from build123d import *

# Parameters (mm, degrees)
SKETCH1_R           = 2.875
SKETCH1_R_2         = 7
BOSS_EXTRUDE1_DEPTH = 24.5875
SKETCH4_W           = 66.272407177
SKETCH4_H           = 27.800260981
CUT_EXTRUDE2_DEPTH  = 20
FILLET3_R           = 10
FILLET4_R           = 10
BOSS_EXTRUDE3_START = -1.5875
BOSS_EXTRUDE3_DEPTH = 1.5875
SKETCH7_R           = 7
CUT_EXTRUDE3_DEPTH  = 1.5875
CUT_EXTRUDE4_START  = -10
SKETCH8_R           = 3
SKETCH8_R_2         = 18.9
SKETCH8_R_3         = 2.875
SKETCH8_R_4         = 7
CUT_EXTRUDE4_DEPTH  = 10
SKETCH9_W           = 229.1070397
SKETCH9_H           = 361.266964835
SKETCH9_R           = 1.388229101
SKETCH9_R_2         = 1.483383261
SKETCH9_R_3         = 1.314910669
SKETCH9_R_4         = 1.248623853
SKETCH9_R_5         = 1.255629307
SKETCH9_R_6         = 1.53911217
CUT_EXTRUDE5_DEPTH  = 13
SKETCH10_W          = 29.988446547
SKETCH10_H          = 5
SKETCH10_H_2        = 5.75
CUT_EXTRUDE6_DEPTH  = 22
SKETCH11_R          = 5.236653548
CUT_EXTRUDE7_DEPTH  = 10
BOSS_EXTRUDE4_START = -1.59
BOSS_EXTRUDE4_DEPTH = 1.59
SKETCH13_R          = 7
CUT_EXTRUDE8_DEPTH  = 41
SKETCH14_W          = 61.491848917
SKETCH14_H          = 35.587491391
CUT_EXTRUDE9_DEPTH  = 20
FILLET5_R           = 10
SKETCH16_W          = 163.723031551
SKETCH16_H          = 22.872070304
CUT_EXTRUDE11_DEPTH = 35
FILLET6_R           = 10
SKETCH17_R          = 1.53911217
SKETCH17_R_2        = 1.255629307
SKETCH17_R_3        = 1.3
SKETCH17_R_4        = 1.314910669
SKETCH17_R_5        = 1.388229101
SKETCH17_R_6        = 1.5
CUT_EXTRUDE12_DEPTH = 42
CUT_EXTRUDE13_START = -30
SKETCH18_R          = 18.9
CUT_EXTRUDE13_DEPTH = 30
SKETCH19_R          = 7
BOSS_EXTRUDE5_DEPTH = 3.175


with BuildPart() as part:
    # Sketch1 → Boss-Extrude1 (new body)
    with BuildSketch(Plane(origin=(0, 0, 0), x_dir=(1, 0, 0), z_dir=(0, 1, 0))):
        with BuildLine():
            Line((42.32729629, 228.6), (10.454309325, 228.6))
            Line((10.454309325, 228.6), (0, 135.362739137))
            Line((0, 135.362739137), (0, 0))
            Line((0, 0), (24.327009544, 0))
            Line((24.327009544, 0), (50.8, 0))
            Line((50.8, 0), (50.8, 64.87909603))
            Line((50.8, 64.87909603), (50.8, 87.423477361))
            Line((50.8, 87.423477361), (50.8, 98.200996728))
            ThreePointArc((50.8, 98.200996728), (50.4, 101.000996728), (50.8, 103.800996728))
            Line((50.8, 103.800996728), (50.8, 104.488200565))
            Line((50.8, 104.488200565), (50.8, 120.619222808))
            Line((50.8, 120.619222808), (50.8, 135.362739137))
            Line((50.8, 135.362739137), (42.32729629, 228.6))
        make_face()
        with Locations(Location((24.101759227, 108.78493524, 0), (0, 0, 270))):
            Circle(SKETCH1_R, mode=Mode.SUBTRACT)
        with Locations(Location((29.504213454, 189.557234372, 0), (0, 0, 270))):
            Circle(SKETCH1_R_2, mode=Mode.SUBTRACT)
    extrude(amount=BOSS_EXTRUDE1_DEPTH)

    # Sketch4 → Cut-Extrude2 (cut)
    with BuildSketch(Plane(origin=(0, 0, -228.6), x_dir=(-1, 0, 0), z_dir=(0, 0, -1))):
        with Locations((-28.174690156, -1.980940155)):
            Rectangle(SKETCH4_W, SKETCH4_H)
    extrude(amount=-CUT_EXTRUDE2_DEPTH, mode=Mode.SUBTRACT)

    # Fillet3
    fillet3_edges = [part.edges().sort_by_distance(p)[0] for p in [
        (44.144746445, 5.959595168, -208.6),
    ]]
    fillet(fillet3_edges, radius=FILLET3_R)

    # Fillet4
    fillet4_edges = [part.edges().sort_by_distance(p)[0] for p in [
        (50.8, 12.29375, 0),
        (0, 12.29375, 0),
        (8.211791854, 5.959595168, -208.6),
    ]]
    fillet(fillet4_edges, radius=FILLET4_R)

    # Sketch6 → Boss-Extrude3 (add)
    with BuildSketch(Plane(origin=(0, 24.5875, 0), x_dir=(1, 0, 0), z_dir=(0, 1, 0)).offset(BOSS_EXTRUDE3_START)):
        with BuildLine():
            Line((50.8, 135.362739137), (50.8, 103.800996728))
            ThreePointArc((50.8, 103.800996728), (50.4, 101.000996728), (50.8, 98.200996728))
            Line((50.8, 98.200996728), (50.8, 61.124243317))
            Line((50.8, 61.124243317), (69.258211507, 96.360728536))
            ThreePointArc((69.258211507, 96.360728536), (70.393157133, 101.370875786), (68.890940865, 106.283413148))
            Line((68.890940865, 106.283413148), (50.8, 135.362739137))
        make_face()
    extrude(amount=BOSS_EXTRUDE3_DEPTH)

    # Sketch7 → Cut-Extrude3 (cut)
    with BuildSketch(Plane(origin=(0, 24.5875, 0), x_dir=(1, 0, 0), z_dir=(0, 1, 0))):
        with Locations(Location((60.4, 101.000996728, 0), (0, 0, 270))):
            Circle(SKETCH7_R)
    extrude(amount=-CUT_EXTRUDE3_DEPTH, mode=Mode.SUBTRACT)

    # Sketch8 → Cut-Extrude4 (cut)
    with BuildSketch(Plane(origin=(0, 24.5875, 0), x_dir=(1, 0, 0), z_dir=(0, 1, 0)).offset(CUT_EXTRUDE4_START)):
        with BuildLine():
            Line((10.454309325, 228.6), (0, 135.362739137))
            Line((0, 135.362739137), (0, 10))
            ThreePointArc((0, 10), (2.928932188, 2.928932188), (10, 0))
            Line((10, 0), (40.8, 0))
            ThreePointArc((40.8, 0), (47.871067812, 2.928932188), (50.8, 10))
            Line((50.8, 10), (50.8, 61.124243317))
            Line((50.8, 61.124243317), (69.258211507, 96.360728536))
            ThreePointArc((69.258211507, 96.360728536), (70.393157133, 101.370875786), (68.890940865, 106.283413148))
            Line((68.890940865, 106.283413148), (50.8, 135.362739137))
            Line((50.8, 135.362739137), (42.32729629, 228.6))
            Line((42.32729629, 228.6), (10.454309325, 228.6))
        make_face()
        with Locations(Location((9.492033273, 118.909935242, 0), (0, 0, 270))):
            Circle(SKETCH8_R, mode=Mode.SUBTRACT)
        with Locations(Location((24.583834565, 64.593886665, 0), (0, 0, 270))):
            Circle(SKETCH8_R_2, mode=Mode.SUBTRACT)
        with Locations(Location((24.101759227, 108.78493524, 0), (0, 0, 270))):
            Circle(SKETCH8_R_3, mode=Mode.SUBTRACT)
        with Locations((60.4, 101.000996728)):
            Circle(SKETCH8_R_4, mode=Mode.SUBTRACT)
        with Locations(Location((29.504213454, 189.557234372, 0), (0, 0, 270))):
            Circle(SKETCH8_R_4, mode=Mode.SUBTRACT)
    extrude(amount=CUT_EXTRUDE4_DEPTH, mode=Mode.SUBTRACT)

    # Sketch9 → Cut-Extrude5 (cut)
    with BuildSketch(Plane.XZ):
        with Locations((19.903204009, -125.752229467)):
            Rectangle(SKETCH9_W, SKETCH9_H)
        with Locations(Location((6.335590122, -44.288799513, 0), (0, 0, 270))):
            Circle(SKETCH9_R, mode=Mode.SUBTRACT)
        with Locations(Location((43.447673368, -42.868436544, 0), (0, 0, 270))):
            Circle(SKETCH9_R_2, mode=Mode.SUBTRACT)
        with Locations(Location((4.659546827, -82.793173401, 0), (0, 0, 270))):
            Circle(SKETCH9_R_3, mode=Mode.SUBTRACT)
        with Locations(Location((48.400988852, -71.551011715, 0), (0, 0, 270))):
            Circle(SKETCH9_R_4, mode=Mode.SUBTRACT)
        with Locations(Location((5.88467603, -135.103145298, 0), (0, 0, 270))):
            Circle(SKETCH9_R_5, mode=Mode.SUBTRACT)
        with Locations(Location((45.747747887, -129.863467374, 0), (0, 0, 270))):
            Circle(SKETCH9_R_6, mode=Mode.SUBTRACT)
    extrude(amount=-CUT_EXTRUDE5_DEPTH, mode=Mode.SUBTRACT)

    # Sketch10 → Cut-Extrude6 (cut)
    with BuildSketch(Plane(origin=(0, 24.5875, 0), x_dir=(1, 0, 0), z_dir=(0, 1, 0))):
        with Locations((23.779803557, 122.41493524)):
            Rectangle(SKETCH10_W, SKETCH10_H)
        with Locations((23.779803557, 108.78493524)):
            Rectangle(SKETCH10_W, SKETCH10_H_2)
        with Locations((23.779803557, 95.528937895)):
            Rectangle(SKETCH10_W, SKETCH10_H)
    extrude(amount=-CUT_EXTRUDE6_DEPTH, mode=Mode.SUBTRACT)

    # Sketch11 → Cut-Extrude7 (cut)
    with BuildSketch(Plane(origin=(0, 24.5875, 0), x_dir=(1, 0, 0), z_dir=(0, 1, 0))):
        with Locations((8.535526315, 118.29502971)):
            Circle(SKETCH11_R)
    extrude(amount=-CUT_EXTRUDE7_DEPTH, mode=Mode.SUBTRACT)

    # Sketch12 → Boss-Extrude4 (add)
    with BuildSketch(Plane(origin=(0, 14.5875, 0), x_dir=(1, 0, 0), z_dir=(0, 1, 0)).offset(BOSS_EXTRUDE4_START)):
        with BuildLine():
            Line((68.287536191, 107.148091395), (50.8, 133.900488173))
            Line((50.8, 133.900488173), (50.8, 103.800996728))
            ThreePointArc((50.8, 103.800996728), (58.520134646, 110.822712782), (68.287536191, 107.148091395))
        make_face()
        with BuildLine():
            Line((69.19540964, 105.759228466), (68.287536191, 107.148091395))
            ThreePointArc((68.287536191, 107.148091395), (58.520134646, 110.822712782), (50.8, 103.800996728))
            ThreePointArc((50.8, 103.800996728), (50.4, 101.000996728), (50.8, 98.200996728))
            ThreePointArc((50.8, 98.200996728), (59.211240578, 91.07190558), (69.067690563, 96.013899345))
            ThreePointArc((69.067690563, 96.013899345), (70.061182785, 98.419999404), (70.4, 101.000996728))
            ThreePointArc((70.4, 101.000996728), (70.094175994, 103.455167016), (69.19540964, 105.759228466))
        make_face()
        with BuildLine():
            ThreePointArc((69.067690563, 96.013899345), (59.211240578, 91.07190558), (50.8, 98.200996728))
            Line((50.8, 98.200996728), (50.8, 64.264230765))
            Line((50.8, 64.264230765), (69.067690563, 96.013899345))
        make_face()
    extrude(amount=BOSS_EXTRUDE4_DEPTH)

    # Sketch13 → Cut-Extrude8 (cut)
    with BuildSketch(Plane(origin=(0, 14.5875, 0), x_dir=(1, 0, 0), z_dir=(0, 1, 0))):
        with Locations(Location((60.4, 101.000996728, 0), (0, 0, 270))):
            Circle(SKETCH13_R)
    extrude(amount=-CUT_EXTRUDE8_DEPTH, mode=Mode.SUBTRACT)

    # Sketch14 → Cut-Extrude9 (cut)
    with BuildSketch(Plane(origin=(0, 0, -228.6), x_dir=(-1, 0, 0), z_dir=(0, 0, -1))):
        with Locations((-33.296946078, 21.381494753)):
            Rectangle(SKETCH14_W, SKETCH14_H)
    extrude(amount=-CUT_EXTRUDE9_DEPTH, mode=Mode.SUBTRACT)

    # Fillet5
    fillet5_edges = [part.edges().sort_by_distance(p)[0] for p in [
        (44.144746445, 13.79375, -208.6),
        (8.211791854, 13.79375, -208.6),
    ]]
    fillet(fillet5_edges, radius=FILLET5_R)

    # Sketch16 → Cut-Extrude11 (cut)
    with BuildSketch(Plane.XY):
        with Locations((6.935844153, 9.456999915)):
            Rectangle(SKETCH16_W, SKETCH16_H)
    extrude(amount=-CUT_EXTRUDE11_DEPTH, mode=Mode.SUBTRACT)

    # Fillet6
    fillet6_edges = [part.edges().sort_by_distance(p)[0] for p in [
        (0, 13.79375, -35),
        (50.8, 13.79375, -35),
    ]]
    fillet(fillet6_edges, radius=FILLET6_R)

    # Sketch17 → Cut-Extrude12 (cut)
    with BuildSketch(Plane.XZ):
        with Locations(Location((45.747747887, -129.863467374, 0), (0, 0, 270))):
            Circle(SKETCH17_R)
        with Locations(Location((5.88467603, -135.103145298, 0), (0, 0, 270))):
            Circle(SKETCH17_R_2)
        with Locations(Location((48.400988852, -71.551011715, 0), (0, 0, 270))):
            Circle(SKETCH17_R_3)
        with Locations(Location((4.659546827, -82.793173401, 0), (0, 0, 270))):
            Circle(SKETCH17_R_4)
        with Locations(Location((6.335590122, -44.288799513, 0), (0, 0, 270))):
            Circle(SKETCH17_R_5)
        with Locations(Location((43.447673368, -42.868436544, 0), (0, 0, 270))):
            Circle(SKETCH17_R_6)
    extrude(amount=-CUT_EXTRUDE12_DEPTH, mode=Mode.SUBTRACT)

    # Sketch18 → Cut-Extrude13 (cut)
    with BuildSketch(Plane(origin=(0, 24.5875, 0), x_dir=(1, 0, 0), z_dir=(0, 1, 0)).offset(CUT_EXTRUDE13_START)):
        with Locations(Location((24.583834565, 64.593886665, 0), (0, 0, 270))):
            Circle(SKETCH18_R)
    extrude(amount=CUT_EXTRUDE13_DEPTH, mode=Mode.SUBTRACT)

    # Sketch19 → Boss-Extrude5 (add)
    # profile 1 of 2: a face of its own
    with BuildSketch(Plane(origin=(0, 14.5875, 0), x_dir=(1, 0, 0), z_dir=(0, 1, 0))):
        Polygon((0, 45), (0, 65), (-40, 65), (-40, 35), (0, 35), align=None)
        with Locations(Location((-20, 50, 0), (0, 0, 270))):
            Circle(SKETCH19_R, mode=Mode.SUBTRACT)
    # profile 2 of 2: a face of its own
    with BuildSketch(Plane(origin=(0, 14.5875, 0), x_dir=(1, 0, 0), z_dir=(0, 1, 0))):
        with BuildLine():
            ThreePointArc((10, 35), (2.928932188, 37.928932188), (0, 45))
            Line((0, 45), (0, 35))
            Line((0, 35), (10, 35))
        make_face()
    extrude(amount=-BOSS_EXTRUDE5_DEPTH)


solid = part.part
CAD build for the part. Positions are in the model's coordinates, mm. A direction names the side the tool comes from. Give positions to 0.01 mm unless a question says otherwise; leave off trailing zeros. Loops run counter-clockwise (first coordinate to the right, second up) from the corner with the lowest first, then second, coordinate; pieces in that order, holes last. Notation, with made-up numbers: M -22.5,36 L 13.5,36 A31 ccw 13.5,73 Z; hole C -32,18.5 d4. An arc over 180 degrees is marked long. One line per question, with ' | ' between items. Start each with the question number.
1. Saw through at C-C on y = 11.9. Give the cut face in (x, z), plus the area to 3 significant figures.
2. Saw through at D-D on z = -50. Give the cut face in (x, y).
3. 3-axis set-ups, long thin cutter, end or side, ignore diameter. For faces 4 (the face through (57.719, 13.804, -94.535)), 5 (the face through (25, 13, -140)): which of +Z, -Z, +X, -X, +Y, -Y reach the whole face in a straight line?
4. Probe L1, parallel to Z at x = 32.5, y = 14.2; L2, parallel to X at y = 13.7, z = -50; L3, parallel to Z at x = -3, y = 13.4. List the from-to ranges inside material, lowest first. Write a range as from..to.
5. Flat gauge pins, fed straight in: pin 1 (1.5 mm diameter, centred on x = 5.88, z = -135.1, fed in from -Y); pin 2 (1.3 mm diameter, centred on y = 14, z = -109.5, fed in from +X); pin 3 (1.3 mm diameter, centred on y = 13.5, z = -57.5, fed in from +X); pin 4 (5 mm diameter, centred on x = 8, z = -151, fed in from -Y). Where does each tip first touch, or does it go through?
6. Saw through at A-A on x = -20. Give the cut face in (y, z).
7. Two-plate mould, pull along X, no slides. Class faces 1 (the face through (3.01, 12.22, -37.85)), 2 (the face through (-20, 13, -65)), 3 (the face through (-22.681, 13.022, -43.534)): pulls with the +X half, pulls with the -X half, needs draft (parallel to the pull), parting line crosses it, or undercut.
Result sheet:
1) outline: M -40,-65 L 0,-65 L 0,-45 A10 cw 10,-35 L -40,-35 Z; hole C -20,-50 d14 | area: 1,070 mm^2
2) outline: M -40,11.41 L -27,11.41 L -27,14.59 L -40,14.59 Z; M -13,11.41 L 0,11.41 L 0,13 L 12.57,13 L 12.57,14.59 L -13,14.59 Z; M 36.59,13 L 50.8,13 L 50.8,14.59 L 36.59,14.59 Z
3) face 4: +Y, -Y | face 5: -Z, +X, -Y
4) L1: z = -208.6..-195.88, -183.23..-124.91, -119.91..-111.66, -105.91..-98.03, -93.03..-81.76, -47.43..-35 | L2: x = -40..-27, -13..12.57, 36.59..50.8 | L3: z = -65..-35
5) pin 1: passes through | pin 2: stops at x = 67.18 | pin 3: stops at x = 50.8 | pin 4: stops at y = 13
6) outline: M 11.41,-65 L 14.59,-65 L 14.59,-57 L 11.41,-57 Z; M 11.41,-43 L 14.59,-43 L 14.59,-35 L 11.41,-35 Z
7) face 1: pulls with the +X half | face 2: needs draft | face 3: undercut
